Autodesk Inventor part; units mm, degrees
ref_plane "end_2_XY" through (-6.3, 10.5, 6.25) normal (0, 1, 0) x (1, 0, 0)
ref_plane "end_2_YZ" through (-6.3, 10.5, 6.25) normal (1, 0, 0) x (0, 0, -1)
ref_plane "end_2_ZX" through (-6.3, 10.5, 6.25) normal (0, 0, -1) x (0, 1, 0)
sketch "Sketch_45" plane through (0, 0, 0) normal (0, 0, 1) x (1, 0, 0)
  arc A0 (2, -9.75) -> (0, -7.75) centre (0, -9.75) ccw
  line L0 (2, -9.75) -> (16, -9.75)
  line L1 (16, -9.75) -> (16, 9.75)
  line L2 (16, 9.75) -> (2, 9.75)
  arc A1 (0, 7.75) -> (2, 9.75) centre (0, 9.75) ccw
  line L3 (0, 7.75) -> (0, -7.75)
  circle A2 centre (12, 0) radius 1.5
  circle A3 centre (4, 0) radius 1.5
extrude "Extrusion1" add sketch "Sketch_45" along normal blind 2
sketch "Sketch_47" plane through (0, 11, 0) normal (0, 1, 0) x (1, 0, 0)
  arc A0 (-6.3, 0) -> (-4.283, -12.1656) centre (-6.3, -6.25) ccw
  line L0 (-4.283, -12.1656) -> (15.3227, -5.4809)
  arc A1 (15.3227, -5.4809) -> (16, -4.5344) centre (15, -4.5344) ccw
  line L1 (16, -4.5344) -> (16, 0)
  line L2 (16, 0) -> (-6.3, 0)
  circle A2 centre (-6.3, -6.25) radius 3
extrude "Extrusion2" add sketch "Sketch_47" against normal blind 1.25
sketch "Sketch_76" plane through (0, -11, 0) normal (0, 1, 0) x (1, 0, 0)
  arc A0 (-6.3, 0) -> (-4.283, -12.1656) centre (-6.3, -6.25) ccw
  line L0 (-4.283, -12.1656) -> (15.3227, -5.4809)
  arc A1 (15.3227, -5.4809) -> (16, -4.5344) centre (15, -4.5344) ccw
  line L1 (16, -4.5344) -> (16, 0)
  line L2 (16, 0) -> (-6.3, 0)
  circle A2 centre (-6.3, -6.25) radius 3
extrude "Extrusion3" add sketch "Sketch_76" along normal blind 1.25
ref_plane "end_2_XY" through (-6.3, 10.5, 6.25) normal (0, 1, 0) x (1, 0, 0)
ref_plane "end_2_YZ" through (-6.3, 10.5, 6.25) normal (1, 0, 0) x (0, 0, -1)
ref_plane "end_2_ZX" through (-6.3, 10.5, 6.25) normal (0, 0, -1) x (0, 1, 0)
ref_plane "end_move_XY" through (-6.3, -11.5, 6.25) normal (0, -1, 0) x (1, 0, 0)
ref_plane "end_move_YZ" through (-6.3, -11.5, 6.25) normal (1, 0, 0) x (0, 0, 1)
ref_plane "end_move_ZX" through (-6.3, -11.5, 6.25) normal (0, 0, 1) x (0, -1, 0)
ref_plane "to_dummy_XY" through (0, 0, 0) normal (0, 0, 1) x (1, 0, 0)
ref_plane "to_dummy_YZ" through (0, 0, 0) normal (1, 0, 0) x (0, 1, 0)
ref_plane "to_dummy_ZX" through (0, 0, 0) normal (0, 1, 0) x (0, 0, 1)
properties part number "045-16-1_se08f"
Could you check a few things on this model? Use its own coordinates, in mm. A direction names the side the tool comes from. Give positions to 0.01 mm unless a question says otherwise; leave off trailing zeros. Order: outer loops, then holes, each group sorted by start corner. A loop starts at its lowest first (then second) coordinate and runs counter-clockwise, first axis right, second up. Notation, with made-up numbers: (79.25, -28.5) - (105.25, -28.5) arc R26 cw to (105.25, 4.5) - close; hole circle Ø8 at (-31.5, 41.5). An arc over 180 degrees is marked (long way). Return JSON: item names as keys, results as strings. Group by question number.
Q1. Suppose I cut it at B-B, the plane z = 8.25. Please give me the cut outline in (x, y), and give its area (3 significant figures).
Q2. Please list where these lines run through material, in increasing order: line 1 along Y through (x, z) = (2.5, 7); line 2 along Y through (x, z) = (4, 0.55); line 3 along Z through (x, y) = (13, 5). Write a range as [from, to].
Q3. Suppose I cut it at D-D, the plane x = 13. Please give me the cut outline in (y, z).
Q4. Thinking about a two-plate mould opening in Z: for faces 5 (the face through (15.82, -10.38, 5.11)), 6 (the face through (-12.49, 10.38, 7.12)), 7 (the face through (2, 11, 5)), 8 (the face through (-3.44, 10.38, 5.35)), which applies, pulls with the +Z half, pulls with the -Z half, needs draft (parallel to the pull), parting line crosses it, or undercut?
Q5. Will these pins go through, and if not, where does the flat tip stop? pin 1 Ø4 at (x, y) = (4, 0) entering from +Z; pin 2 Ø1.8 at (x, y) = (12, 0) entering from +Z; pin 3 Ø1.6 at (y, z) = (-2, 1) entering from -X.
Q6. Suppose I cut it at C-C, the plane z = 1.5. Please give me the cut outline in (x, y).
Q7. Which directions (+Z, -Z, +X, -X, +Y, -Y) give clear straight access to the entire face, cutting with the end or side of a thin tool? Please do faces 1 (the face through (-2, 9.75, 6)), 2 (the face through (8, 0, 2)), 3 (the face through (5.386, 0.575, 0.986)), 4 (the face through (1.43, 8.35, 0.99)).
Q8. Suppose I cut it at A-A, the plane y = 0. Please give me the cut outline in (x, z).
Resolved:
{
 "1": {"outline": "(-12.22, -11) - (-8.54, -11) - (-8.54, -9.75) - (-12.22, -9.75) - close; (-12.22, 9.75) - (-8.54, 9.75) - (-8.54, 11) - (-12.22, 11) - close; (-4.06, -11) - (7.2, -11) - (7.2, -9.75) - (-4.06, -9.75) - close; (-4.06, 9.75) - (7.2, 9.75) - (7.2, 11) - (-4.06, 11) - close", "area": "37.4 mm2"},
 "2": {"line 1": "y = [-11, -9.75], [9.75, 11]", "line 2": "y = [-11, -1.5], [1.5, 11]", "line 3": "z = [0, 2]"},
 "3": {"outline": "(-11, 0) - (-1.12, 0) - (-1.12, 2) - (-9.75, 2) - (-9.75, 6.27) - (-11, 6.27) - close; (1.12, 0) - (11, 0) - (11, 6.27) - (9.75, 6.27) - (9.75, 2) - (1.12, 2) - close"},
 "4": {"face 5": "pulls with the +Z half", "face 6": "parting line crosses it", "face 7": "needs draft", "face 8": "undercut"},
 "5": {"pin 1": "stops at z = 2", "pin 2": "passes through", "pin 3": "stops at x = 0"},
 "6": {"outline": "(-10.36, -11) - (16, -11) - (16, 11) - (-10.36, 11) - (-10.36, 9.75) - (2, 9.75) arc R2 cw to (0, 7.75) - (0, -7.75) arc R2 cw to (2, -9.75) - (-10.36, -9.75) - close; hole circle Ø3 at (4, 0); hole circle Ø3 at (12, 0)"},
 "7": {"face 1": "+Z, -X", "face 2": "+Z, +X, -X", "face 3": "+Z, -Z", "face 4": "+Z, -Z, -X"},
 "8": {"outline": "(0, 0) - (2.5, 0) - (2.5, 2) - (0, 2) - close; (5.5, 0) - (10.5, 0) - (10.5, 2) - (5.5, 2) - close; (13.5, 0) - (16, 0) - (16, 2) - (13.5, 2) - close"}
}
